Part model, mm, in its own coordinate system. Give positions to 0.01 mm unless a question says otherwise; leave off trailing zeros. Order: outer loops, then holes, each group sorted by start corner. A loop starts at its lowest first (then second) coordinate and runs counter-clockwise, first axis right, second up. Notation, with made-up numbers: (28.25, 47.5) -> (83.25, 47.5) arc R21 ccw to (83.25, 82.5) -> close; hole circle Ø3 at (35, -20). An arc over 180 degrees is marked (long way). Write item = value, one per line. Start each with the question number.
(1) Flat gauge pins, fed straight in: pin 1 (0.9 mm diameter, centred on x = 203, y = 1.5, fed in from +Z); pin 2 (0.9 mm diameter, centred on x = 297, y = 2, fed in from -Z); pin 3 (5 mm diameter, centred on x = 284.25, z = -137.25, fed in from +Y); pin 4 (1.5 mm diameter, centred on x = 190, y = 2, fed in from -Z). Where does each tip first touch, or does it go through?
(2) Saw through at A-A, the plane y = 1.1. State how many separate pieces and enclosed holes the cut face has, then the cut area to 3 significant figures.
(3) Saw through at C-C, the plane x = 274.5. List the corners of the cut face in (y, z), then the cut area to 3 significant figures.
(4) Probe line 1 along X through (y, z) = (2.3, -137.25); line 2 along X through (y, z) = (1.5, -168.75); line 3 along Z through (x, y) = (253.75, 2.4). List the from-to ranges inside material, lowest first. Write a range as from..to.
(5) Saw through at B-B, the plane z = -100. List the corners of the cut face in (x, y).
from build123d import *

# Parameters (mm, degrees)
SKETCH1_R           = 1.6
BOSS_EXTRUDE1_DEPTH = 3


with BuildPart() as part:
    # Sketch1 → Boss-Extrude1 (new body)
    with BuildSketch(Plane(origin=(0, 0, 0), x_dir=(1, 0, 0), z_dir=(0, 1, 0))):
        Polygon((0, 0), (0, 40), (-3, 40), (-3, 70), (0, 70), (0, 187), (-3, 187), (-3, 217), (0, 217), (0, 334), (-3, 334), (-3, 364), (0, 364), (0, 404), (30, 404), (30, 407), (60, 407), (60, 404), (140, 404), (140, 407), (170, 407), (170, 404), (200, 404), (214.29020853, 390.007504148), (216.389082908, 392.151035427), (237.824395702, 371.162291649), (235.725521325, 369.01876037), (260.274478675, 344.98123963), (262.373353053, 347.12477091), (283.808665848, 326.136027132), (281.70979147, 323.992495852), (296, 310), (296, 270), (299, 270), (299, 240), (296, 240), (296, 170), (299, 170), (299, 140), (296, 140), (296, 70), (299, 70), (299, 40), (296, 40), (296, 0), (256, 0), (256, -3), (226, -3), (226, 0), (163, 0), (163, -3), (133, -3), (133, 0), (70, 0), (70, -3), (40, -3), (40, 0), align=None)
        with Locations(Location((253.75, 168.75, 0), (0, 0, 270))):
            Circle(SKETCH1_R, mode=Mode.SUBTRACT)
        with Locations(Location((284.25, 168.75, 0), (0, 0, 270))):
            Circle(SKETCH1_R, mode=Mode.SUBTRACT)
        with Locations(Location((284.25, 137.25, 0), (0, 0, 270))):
            Circle(SKETCH1_R, mode=Mode.SUBTRACT)
        with Locations(Location((253.75, 137.25, 0), (0, 0, 270))):
            Circle(SKETCH1_R, mode=Mode.SUBTRACT)
    extrude(amount=BOSS_EXTRUDE1_DEPTH)


solid = part.part
Results list:
q1.pin_1 = 0
q1.pin_2 = -270
q1.pin_3 = 3
q1.pin_4 = -404
q2.separate_pieces = 1
q2.enclosed_holes = 4
q2.area = 116,000 mm^2
q3.outline = (0, -335.25) -> (3, -335.25) -> (3, 0) -> (0, 0) -> close
q3.area = 1,010 mm^2
q4.line_1 = 0..252.15, 255.35..282.65, 285.85..296
q4.line_2 = 0..252.15, 255.35..282.65, 285.85..299
q4.line_3 = -351.37..-170.35, -167.15..-138.85, -135.65..3
q5.outline = (0, 0) -> (296, 0) -> (296, 3) -> (0, 3) -> close
